Geometry check sheet. Reference: drawing and pictorial views, mm from the part's lowest x, y, z. A direction names the side the tool comes from. Give positions to 0.01 mm unless a question says otherwise; leave off trailing zeros. Order: outer loops, then holes, each group sorted by start corner. A loop starts at its lowest first (then second) coordinate and runs counter-clockwise, first axis right, second up. Notation, with made-up numbers: M 64.25,41.25 L 74.25,41.25 A20 cw 74.25,73.25 Z; hole C 7.25,20.25 d7. An arc over 180 degrees is marked long. Answer as a JSON object with one key per item and string values. Group by question number.
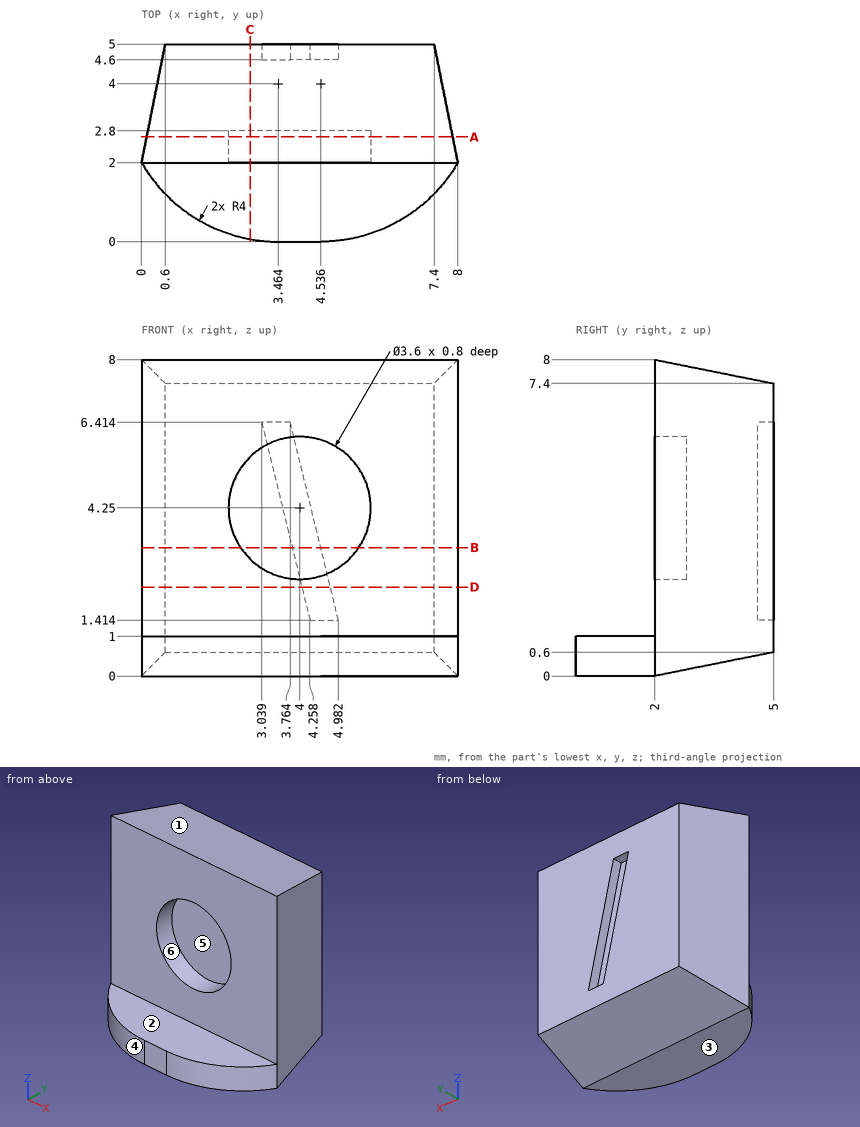
1. Cross-section at A-A (y = 2.65). Record the cut outline in (x, z).
2. Thickness scan on line 1 along X through (y, z) = (2.35, 4.25); line 2 along Z through (x, y) = (5, 1.85); line 3 along Y through (x, z) = (2.5, 4). Record the ranges inside material, lowest first. Write a range as [from, to].
3. Access from +Z, -Z, +X, -X, +Y, -Y to the whole of each face (thin tool, end or side, straight path). Record for the marked faces 1 and 2.
4. Release check for a two-part mould opening along Z. For the marked faces 3, 4, 5 and 6 record: released by +Z, released by -Z, zero draft, split by the parting line, or undercut.
5. Depth check by flat-ended pin: pin 1 (4.5 mm diameter, centred on x = 4, z = 4.25, fed in from -Y); pin 2 (1 mm diameter, centred on x = 3.5, y = 1, fed in from +Z). Enter the tip coordinate at first touch or a pass-through.
6. Cross-section at D-D (z = 2.25). Record the cut outline in (x, y) (1 decimal), and give its area (3 significant figures).
7. Cross-section at C-C (x = 2.75). Record the cut outline in (y, z) (1 decimal).
8. Cross-section at B-B (z = 3.25). Record the cut outline in (x, y) (1 decimal), and give its area (3 significant figures).
Report:
{
 "1": {"outline": "M 0.13,0.13 L 7.87,0.13 L 7.87,7.87 L 0.13,7.87 Z; hole C 4,4.25 d3.6"},
 "2": {"line 1": "x = [0.07, 2.2], [5.8, 7.93]", "line 2": "z = [0, 1]", "line 3": "y = [2.8, 5]"},
 "3": {"face 1": "+Z, +X, -X, +Y", "face 2": "+Z, +X, -X, -Y"},
 "4": {"face 3": "released by -Z", "face 4": "zero draft", "face 5": "undercut", "face 6": "undercut"},
 "5": {"pin 1": "stops at y = 2", "pin 2": "stops at z = 1"},
 "6": {"outline": "M 0,2 L 8,2 L 7.4,5 L 4.8,5 L 4.8,4.6 L 4.1,4.6 L 4.1,5 L 0.6,5 Z", "area": "21.9 mm2"},
 "7": {"outline": "M 0.1,0 L 2,0 L 5,0.6 L 5,7.4 L 2,8 L 2,5.5 L 2.8,5.5 L 2.8,3 L 2,3 L 2,1 L 0.1,1 Z"},
 "8": {"outline": "M 0,2 L 2.5,2 L 2.5,2.8 L 5.5,2.8 L 5.5,2 L 8,2 L 7.4,5 L 4.5,5 L 4.5,4.6 L 3.8,4.6 L 3.8,5 L 0.6,5 Z", "area": "19.5 mm2"}
}
